from build123d import *

# Parameters (mm, degrees)
F0_W      = 33.27621
F0_H      = 40.005
F1_DEPTH  = 45.212
F0_W_2    = 10.9982
F2_DEPTH  = 20.32
F3_SIZE   = 5.0038
F4_R      = 7.62
F5_DEPTH  = 62.738
F6_R      = 2.5019
F7_DEPTH  = 16.764
F8_SIZE   = 0.762
F9_SIZE   = 0.762
F10_W     = 9.116596
F10_H     = 15.0622
F11_DEPTH = 3.048


with BuildPart() as f1:
    # F0 (on Top) → F1 (new body)
    with BuildSketch(Plane.XY):
        Rectangle(F0_W, F0_H)
    extrude(amount=F1_DEPTH)

    # F0 (on Top) → F2 (join)
    with BuildSketch(Plane.XY):
        with Locations((-22.137205, 0)):
            Rectangle(F0_W_2, F0_H)
        with Locations((22.137205, 0)):
            Rectangle(F0_W_2, F0_H)
    extrude(amount=F2_DEPTH)

    # F3
    f3_edges = [f1.edges().sort_by_distance(p)[0] for p in [
        (0, -20.0025, 45.212),
    ]]
    chamfer(f3_edges, length=F3_SIZE)

    # F4 (on Top) → F5 (cut)
    with BuildSketch(Plane.XY):
        with Locations((0, -11.22532)):
            Circle(F4_R)
    extrude(amount=F5_DEPTH, mode=Mode.SUBTRACT)

    # F6 (on Right) → F7 (join, symmetric)
    with BuildSketch(Plane.YZ):
        with Locations((-10.78459, 38.329016)):
            Circle(F6_R)
    extrude(amount=F7_DEPTH, both=True)

    # F8
    f8_edges = [f1.edges().sort_by_distance(p)[0] for p in [
        (-27.636305, 0, 20.32),
    ]]
    chamfer(f8_edges, length=F8_SIZE)

    # F9
    f9_edges = [f1.edges().sort_by_distance(p)[0] for p in [
        (27.636305, 0, 20.32),
    ]]
    chamfer(f9_edges, length=F9_SIZE)

    # F10 (on face) → F11 (cut)
    with BuildSketch(Plane.XZ.offset(20.0025)):
        with Locations((-0.019252, 34.627516)):
            Rectangle(F10_W, F10_H)
    extrude(amount=-F11_DEPTH, mode=Mode.SUBTRACT)


solid = f1.part
Check sheet for the modelled part. Datum: model origin and axes. Units: mm. A direction names the side the tool comes from. Give positions to 0.01 mm unless a question says otherwise; leave off trailing zeros. Write each loop counter-clockwise with the first axis right and the second up, starting at its lowest first coordinate (ties: lowest second). Pieces come first, ordered by that corner, then holes. Notation, with made-up numbers: (-20, 8) -> (32, 8) arc R15 cw to (32, 23) -> close; hole circle Ø7 at (-2, -0.5). An arc over 180 degrees is marked (long way). One line per item, written item: value. Start each with the question number.
Item 1: Section check A-A on z = 30. Record the cut outline in (x, y), then the cut area to 3 significant figures.
Item 2: Draft check along Z on faces 1 (the flat face through (-4.578, -19, 35)), 2 (the flat face through (-11.577, -17.536, 42.675)), 3 (the cylindrical face through (0.1, -9.63, 36.11)), 4 (the flat face through (27.636, 0, 10)). Enter one of: +Z half, -Z half, draft (parallel to the pull), parting line (faces both ways), or undercut.
Item 3: Section check D-D on z = 6. Record the cut outline in (x, y).
Item 4: Section check B-B on y = 0. Record the cut outline in (x, z).
Item 5: Section check C-C on x = 0. Record the cut outline in (y, z), then the cut area to 3 significant figures.
Item 6: Material ranges on probe 1 along X at (y, z) = (-18, 38.5); probe 2 along Y at (x, z) = (0, 18); probe 3 along X at (y, z) = (-2.5, 29.5), recorded low to high. Write a range as from..to.
Item 7: Tool access check on faces 5 (the flat face through (11.391, -17.536, 42.675)), 6 (the flat face through (16.764, -11, 38)), 7 (the flat face through (-16.764, -11, 38)). Record the directions out of +Z, -Z, +X, -X, +Y, -Y that give a thin tool (end or side, any length) a straight path to the whole face; none if there is none.
Item 8: Gauge pin test, flat ends, axial feed: pin 1 (6 mm diameter, centred on y = -9.5, z = 23, fed in from -X); pin 2 (1.5 mm diameter, centred on y = -10.5, z = 38, fed in from +X); pin 3 (8 mm diameter, centred on x = 22, y = -9, fed in from +Z). Record the tip position at first contact, or that the pin passes through.
Results list:
1. outline: (-16.64, -20) -> (-4.58, -20) -> (-4.58, -17.32) arc R7.62 cw (long way) to (4.54, -17.35) -> (4.54, -20) -> (16.64, -20) -> (16.64, 20) -> (-16.64, 20) -> close
1. area: 1,130 mm²
2. face 1: undercut
2. face 2: +Z half
2. face 3: parting line
2. face 4: draft
3. outline: (-27.64, -20) -> (27.64, -20) -> (27.64, 20) -> (-27.64, 20) -> close; hole circle Ø15.24 at (0, -11.23)
4. outline: (-27.64, 0) -> (27.64, 0) -> (27.64, 19.56) -> (26.87, 20.32) -> (16.64, 20.32) -> (16.64, 45.21) -> (-16.64, 45.21) -> (-16.64, 20.32) -> (-26.87, 20.32) -> (-27.64, 19.56) -> close
5. outline: (-20, 0) -> (-18.85, 0) -> (-18.85, 27.1) -> (-20, 27.1) -> close; circle Ø5 at (-10.78, 38.33); (-3.61, 0) -> (20, 0) -> (20, 45.21) -> (-3.61, 45.21) -> close
5. area: 1,120 mm²
6. probe 1: -16.64..-4.58, 4.54..16.64
6. probe 2: -20..-18.85, -3.61..20
6. probe 3: -16.64..16.64
7. face 5: +Z, +X, -X, -Y
7. face 6: +Z, +X, +Y, -Y
7. face 7: +Z, -X, +Y, -Y
8. pin 1: x = -27.19
8. pin 2: x = 16.76
8. pin 3: z = 20.32
